Can you work these out from the model? Positions are in its coordinate system, mm. A direction names the side the tool comes from. Give positions to 0.01 mm unless a question says otherwise; leave off trailing zeros. Write each loop counter-clockwise with the first axis right and the second up, starting at its lowest first coordinate (ties: lowest second). Pieces come first, ordered by that corner, then holes. Notation, with made-up numbers: M -2.5,71 L 29.5,71 A12 ccw 29.5,90 Z; hole C -36,25 d9. An arc over 180 degrees is marked long. Write each question's results on one line, items separated by ' | '.
Autodesk Inventor part; units mm, degrees
ref_plane "YZ Plane" through (0, 0, 0) normal (1, 0, 0) x (0, 1, 0)
ref_plane "XZ Plane" through (0, 0, 0) normal (0, 1, 0) x (-1, 0, 0)
ref_plane "XY Plane" through (0, 0, 0) normal (0, 0, 1) x (1, 0, 0)
sketch "Sketch1" plane through (0, 0, 0) normal (1, 0, 0) x (0, 1, 0)
  circle A0 centre (0, 0) radius 15
  dimension "d0" = 30
extrude "Extrusion1" add sketch "Sketch1" along normal mid plane 120
sketch "Sketch2" plane through (60, 0, 0) normal (1, 0, 0) x (0, 0, -1)
  line L0 (-17.5, 17.5) -> (17.5, 17.5)
  line L1 (17.5, 17.5) -> (17.5, -17.5)
  line L2 (17.5, -17.5) -> (-17.5, -17.5)
  line L3 (-17.5, -17.5) -> (-17.5, 17.5)
  line L4 (-17.5, 17.5) -> (17.5, -17.5) construction
  line L5 (17.5, 17.5) -> (-17.5, -17.5) construction
  point P0 (0, 0)
  dimension "d3" = 35
  dimension "d4" = 35
extrude "Extrusion2" add sketch "Sketch2" along normal blind 20
mirror "Mirror1" about plane through (0, 0, 0) normal (1, 0, 0) of "Extrusion2"
properties part number "ROLLER SHAFT"
Item 1: For faces 1 (the face through (70, 0, 17.5)), 2 (the face through (0.84, -14.985, 0.66)), which set-ups out of +Z, -Z, +X, -X, +Y, -Y let a thin tool reach every point of the face, with its end or its side?
Geometry says:
face 1: +Z, +X, -X, +Y, -Y | face 2: none
Item 2: If I drill on line 1 (X direction, y = -10, z = 13.5); line 2 (Z direction, x = 42.5, y = 0); line 3 (Y direction, x = -17, z = -12), over which ranges is the centre line in solid material (lowest first)? Write a range as from..to.
Geometry says:
line 1: x = -80..-60, 60..80 | line 2: z = -15..15 | line 3: y = -9..9
Item 3: I want a section at C-C, the plane x = -15. Please give me the cut outline in (y, z), and give its area (3 significant figures).
Geometry says:
outline: C 0,0 d30 | area: 707 mm2
Item 4: I'm going to push flat-ended pins straight in: pin 1 (12 mm diameter, centred on x = 41, y = -12.5, fed in from -Z); pin 2 (4 mm diameter, centred on x = -39, z = 12, fed in from -Y); pin 3 (4 mm diameter, centred on x = 12, y = 3, fed in from -Z). Where does each tip first touch, or does it pass through?
Geometry says:
pin 1: stops at z = -13.52 | pin 2: stops at y = -11.18 | pin 3: stops at z = -14.97
Item 5: I want a section at A-A, the plane z = 0. Please give me the cut outline in (x, y), and give its area (3 significant figures).
Geometry says:
outline: M -80,-17.5 L -60,-17.5 L -60,-15 L 60,-15 L 60,-17.5 L 80,-17.5 L 80,17.5 L 60,17.5 L 60,15 L -60,15 L -60,17.5 L -80,17.5 Z | area: 5,000 mm2
Item 6: Thinking about a two-plate mould opening in X: for faces 3 (the face through (-60, 0.2, 15.3)), 4 (the face through (-80, 0, 0)), 5 (the face through (-70, 0, -17.5)), 6 (the face through (80, 0, 0)), which applies, +X half, -X half, draft (parallel to the pull), parting line (faces both ways), or undercut?
Geometry says:
face 3: undercut | face 4: -X half | face 5: draft | face 6: +X half
